```python
from build123d import *

# Parameters (mm, degrees)
BOSS_EXTRU_1_DEPTH      = 5
ESQUISSE2_R             = 13
ESQUISSE2_R_2           = 10
ENL_V_MAT_EXTRU_1_DEPTH = 85.791446444


with BuildPart() as part:
    # Esquisse1 → Boss.-Extru.1 (new body)
    with BuildSketch(Plane.XY):
        with BuildLine():
            Line((-7.756063007, 57.713945373), (-3.353460657, 55.024630504))
            ThreePointArc((-3.353460657, 55.024630504), (0, 54), (3.353460657, 55.024630504))
            Line((3.353460657, 55.024630504), (7.756063007, 57.713945373))
            ThreePointArc((7.756063007, 57.713945373), (10.013220978, 58.695868578), (12.474701449, 58.688856044))
            ThreePointArc((12.474701449, 58.688856044), (14.726228007, 57.694088008), (16.388860271, 55.878987669))
            Line((16.388860271, 55.878987669), (19.316994747, 51.631476586))
            ThreePointArc((19.316994747, 51.631476586), (21.963778726, 49.331454713), (25.444072249, 48.903525925))
            Line((25.444072249, 48.903525925), (30.559892529, 49.569637607))
            ThreePointArc((30.559892529, 49.569637607), (33.021293088, 49.548600235), (35.267115138, 48.541019662))
            ThreePointArc((35.267115138, 48.541019662), (36.919378386, 46.716475488), (37.700000719, 44.382045352))
            Line((37.700000719, 44.382045352), (38.64736627, 39.310771309))
            ThreePointArc((38.64736627, 39.310771309), (40.129820576, 36.133052743), (43.135172596, 34.326557439))
            Line((43.135172596, 34.326557439), (48.079639004, 32.854289173))
            ThreePointArc((48.079639004, 32.854289173), (50.319683635, 31.833928776), (51.961524227, 30))
            ThreePointArc((51.961524227, 30), (52.72883284, 27.66115995), (52.49246855, 25.211044196))
            Line((52.49246855, 25.211044196), (51.295257065, 20.192876545))
            ThreePointArc((51.295257065, 20.192876545), (51.35705188, 16.686917696), (53.367809731, 13.814215325))
            Line((53.367809731, 13.814215325), (57.285979107, 10.45813567))
            ThreePointArc((57.285979107, 10.45813567), (58.917343741, 8.61488183), (59.671313722, 6.271707796))
            ThreePointArc((59.671313722, 6.271707796), (59.420993069, 3.822978563), (58.208511689, 1.680824463))
            Line((58.208511689, 1.680824463), (55.07373191, -2.416550019))
            ThreePointArc((55.07373191, -2.416550019), (53.70418235, -5.644537016), (54.372667732, -9.086730118))
            Line((54.372667732, -9.086730118), (56.587052995, -13.746324501))
            ThreePointArc((56.587052995, -13.746324501), (57.327659867, -16.093756448), (57.063390978, -18.541019662))
            ThreePointArc((57.063390978, -18.541019662), (55.838723774, -20.676230548), (53.859774349, -22.14002509))
            Line((53.859774349, -22.14002509), (49.329458179, -24.608133132))
            ThreePointArc((49.329458179, -24.608133132), (46.765371804, -27), (45.975997522, -30.416497372))
            Line((45.975997522, -30.416497372), (46.103711342, -35.573920284))
            ThreePointArc((46.103711342, -35.573920284), (45.825502796, -38.019638029), (44.588689529, -40.147836382))
            ThreePointArc((44.588689529, -40.147836382), (42.60143186, -41.60033156), (40.198192724, -42.132663168))
            Line((40.198192724, -42.132663168), (35.055672985, -42.544746469))
            ThreePointArc((35.055672985, -42.544746469), (31.740403624, -43.686917696), (29.629659661, -46.486975906))
            Line((29.629659661, -46.486975906), (27.64861916, -51.25046207))
            ThreePointArc((27.64861916, -51.25046207), (26.399699981, -53.371578798), (24.404198585, -54.812727459))
            ThreePointArc((24.404198585, -54.812727459), (21.997965355, -55.331357318), (19.585978387, -54.840181022))
            Line((19.585978387, -54.840181022), (14.720443461, -53.124986634))
            ThreePointArc((14.720443461, -53.124986634), (11.227231304, -52.81997044), (8.160084469, -54.519433984))
            Line((8.160084469, -54.519433984), (4.412829545, -58.065333369))
            ThreePointArc((4.412829545, -58.065333369), (2.409149205, -59.495088726), (0, -60))
            ThreePointArc((0, -60), (-2.409149205, -59.495088726), (-4.412829545, -58.065333369))
            Line((-4.412829545, -58.065333369), (-8.160084469, -54.519433984))
            ThreePointArc((-8.160084469, -54.519433984), (-11.227231304, -52.81997044), (-14.720443461, -53.124986634))
            Line((-14.720443461, -53.124986634), (-19.585978387, -54.840181022))
            ThreePointArc((-19.585978387, -54.840181022), (-21.997965355, -55.331357318), (-24.404198585, -54.812727459))
            ThreePointArc((-24.404198585, -54.812727459), (-26.399699981, -53.371578798), (-27.64861916, -51.25046207))
            Line((-27.64861916, -51.25046207), (-29.629659661, -46.486975906))
            ThreePointArc((-29.629659661, -46.486975906), (-31.740403624, -43.686917696), (-35.055672985, -42.544746469))
            Line((-35.055672985, -42.544746469), (-40.198192724, -42.132663168))
            ThreePointArc((-40.198192724, -42.132663168), (-42.60143186, -41.60033156), (-44.588689529, -40.147836382))
            ThreePointArc((-44.588689529, -40.147836382), (-45.825502796, -38.019638029), (-46.103711342, -35.573920284))
            Line((-46.103711342, -35.573920284), (-45.975997522, -30.416497372))
            ThreePointArc((-45.975997522, -30.416497372), (-46.765371804, -27), (-49.329458179, -24.608133132))
            Line((-49.329458179, -24.608133132), (-53.859774349, -22.14002509))
            ThreePointArc((-53.859774349, -22.14002509), (-55.838723774, -20.676230548), (-57.063390978, -18.541019662))
            ThreePointArc((-57.063390978, -18.541019662), (-57.327659867, -16.093756448), (-56.587052995, -13.746324501))
            Line((-56.587052995, -13.746324501), (-54.372667732, -9.086730118))
            ThreePointArc((-54.372667732, -9.086730118), (-53.70418235, -5.644537016), (-55.07373191, -2.416550019))
            Line((-55.07373191, -2.416550019), (-58.208511689, 1.680824463))
            ThreePointArc((-58.208511689, 1.680824463), (-59.420993069, 3.822978563), (-59.671313722, 6.271707796))
            ThreePointArc((-59.671313722, 6.271707796), (-58.917343741, 8.61488183), (-57.285979107, 10.45813567))
            Line((-57.285979107, 10.45813567), (-53.367809731, 13.814215325))
            ThreePointArc((-53.367809731, 13.814215325), (-51.35705188, 16.686917696), (-51.295257065, 20.192876545))
            Line((-51.295257065, 20.192876545), (-52.49246855, 25.211044196))
            ThreePointArc((-52.49246855, 25.211044196), (-52.72883284, 27.66115995), (-51.961524227, 30))
            ThreePointArc((-51.961524227, 30), (-50.319683635, 31.833928776), (-48.079639004, 32.854289173))
            Line((-48.079639004, 32.854289173), (-43.135172596, 34.326557439))
            ThreePointArc((-43.135172596, 34.326557439), (-40.129820576, 36.133052743), (-38.64736627, 39.310771309))
            Line((-38.64736627, 39.310771309), (-37.700000719, 44.382045352))
            ThreePointArc((-37.700000719, 44.382045352), (-36.919378386, 46.716475488), (-35.267115138, 48.541019662))
            ThreePointArc((-35.267115138, 48.541019662), (-33.021293088, 49.548600235), (-30.559892529, 49.569637607))
            Line((-30.559892529, 49.569637607), (-25.444072249, 48.903525925))
            ThreePointArc((-25.444072249, 48.903525925), (-21.963778726, 49.331454713), (-19.316994747, 51.631476586))
            Line((-19.316994747, 51.631476586), (-16.388860271, 55.878987669))
            ThreePointArc((-16.388860271, 55.878987669), (-14.726228007, 57.694088008), (-12.474701449, 58.688856044))
            ThreePointArc((-12.474701449, 58.688856044), (-10.013220978, 58.695868578), (-7.756063007, 57.713945373))
        make_face()
    extrude(amount=BOSS_EXTRU_1_DEPTH)

    # Esquisse2 → Enlèv. mat.-Extru.1 (cut, through all)
    with BuildSketch(Plane(origin=(0, 0, 0), x_dir=(-1, 0, 0), z_dir=(0, 0, -1))):
        Circle(ESQUISSE2_R)
        with Locations((0, 42)):
            Circle(ESQUISSE2_R_2)
        with Locations((29.69848481, 29.69848481)):
            Circle(ESQUISSE2_R_2)
        with Locations((42, 0)):
            Circle(ESQUISSE2_R_2)
        with Locations((29.69848481, -29.69848481)):
            Circle(ESQUISSE2_R_2)
        with Locations((0, -42)):
            Circle(ESQUISSE2_R_2)
        with Locations((-29.69848481, -29.69848481)):
            Circle(ESQUISSE2_R_2)
        with Locations((-42, 0)):
            Circle(ESQUISSE2_R_2)
        with Locations((-29.69848481, 29.69848481)):
            Circle(ESQUISSE2_R_2)
    extrude(amount=-ENL_V_MAT_EXTRU_1_DEPTH, mode=Mode.SUBTRACT)


solid = part.part
```
Geometry check sheet. Reference: the model listing, model coordinates, mm. A direction names the side the tool comes from. Coordinates: 2 decimals unless noted, no trailing zeros. Order: outer loops, then holes, each group sorted by start corner. A loop starts at its lowest first (then second) coordinate and runs counter-clockwise, first axis right, second up. Notation, with made-up numbers: (-34.75, -4) - (-14.75, -4) arc R22 cw to (-14.75, 10) - close; hole circle Ø1 at (43.5, -35). An arc over 180 degrees is marked (long way). Answer as a JSON object with one key per item and string values. Group by question number.
Item 1: Sectioned sample at B-B, the plane y = 37.5. Record the cut outline in (x, z).
Item 2: Scan lines: probe 1 along Y at (x, z) = (0, 3.25); probe 2 along X at (y, z) = (-29, 4.75); probe 3 along X at (y, z) = (-4, 1.1). Record each from-to range of solid material in increasing order.
Item 3: Sectioned sample at C-C, the plane z = 2.8. Give the number of separate pieces and of enclosed holes in the cut face, and give its area (3 significant figures).
Item 4: Sectioned sample at A-A, the plane x = -33.5. Record the cut outline in (y, z).
Item 5: Tool access check on faces 4 (the face through (6.31, -56.27, 2.46)), 5 (the face through (-28.04, 49.24, 2.46)), 6 (the face through (0.8, 13.4, 0)). Record the directions out of +Z, -Z, +X, -X, +Y, -Y that give a thin tool (end or side, any length) a straight path to the whole face; none if there is none.
Item 6: Depth check by flat-ended pin: pin 1 Ø8 at (x, y) = (33, 13) entering from -Z; pin 2 Ø3 at (y, z) = (18, 3) entering from +X; pin 3 Ø1 at (y, z) = (-37.5, 4) entering from +X. Enter the tip coordinate at first touch or a pass-through.
Item 7: Draft check along Y on faces 1 (the face through (21.92, 49.35, 2.46)), 2 (the face through (51.902, 22.737, 2.465)), 3 (the face through (-37.59, -42.34, 2.46)). Enter one of: +Y half, -Y half, draft (parallel to the pull), parting line (faces both ways), or undercut.
Resolved:
{
 "1": {"outline": "(-39.2, 0) - (-35.95, 0) - (-35.95, 5) - (-39.2, 5) - close; (-23.44, 0) - (-8.93, 0) - (-8.93, 5) - (-23.44, 5) - close; (8.93, 0) - (23.44, 0) - (23.44, 5) - (8.93, 5) - close; (35.95, 0) - (39.2, 0) - (39.2, 5) - (35.95, 5) - close"},
 "2": {"probe 1": "-60 to -52, -32 to -13, 13 to 32, 52 to 54", "probe 2": "-46.05 to -39.67, -19.72 to 19.72, 39.67 to 46.05", "probe 3": "-54.12 to -51.17, -32.83 to -12.37, 12.37 to 32.83, 51.17 to 54.12"},
 "3": {"separate pieces": "1", "enclosed holes": "9", "area": "7,170 mm^2"},
 "4": {"outline": "(-42.81, 0) - (-38.95, 0) - (-38.95, 5) - (-42.81, 5) - close; (-20.45, 0) - (-5.27, 0) - (-5.27, 5) - (-20.45, 5) - close; (5.27, 0) - (20.45, 0) - (20.45, 5) - (5.27, 5) - close; (38.95, 0) - (49.42, 0) - (49.42, 5) - (38.95, 5) - close"},
 "5": {"face 4": "+Z, -Z, -Y", "face 5": "+Z, -Z, +Y", "face 6": "-Z, +X, -X, +Y, -Y"},
 "6": {"pin 1": "z = 0", "pin 2": "x = 51.42", "pin 3": "x = 46.07"},
 "7": {"face 1": "+Y half", "face 2": "undercut", "face 3": "-Y half"}
}
